Job drawing, mm, ordinate dimensions from the low corner. One solid piece. Give positions to 0.01 mm unless a question says otherwise; leave off trailing zeros. Loops run counter-clockwise (first coordinate to the right, second up) from the corner with the lowest first, then second, coordinate; pieces in that order, holes last. Notation, with made-up numbers: M 30,26.25 L 53,26.25 A8 cw 53,39.25 Z; hole C -12,-1 d2. An arc over 180 degrees is marked long. Answer in a Markdown table with one row per item.
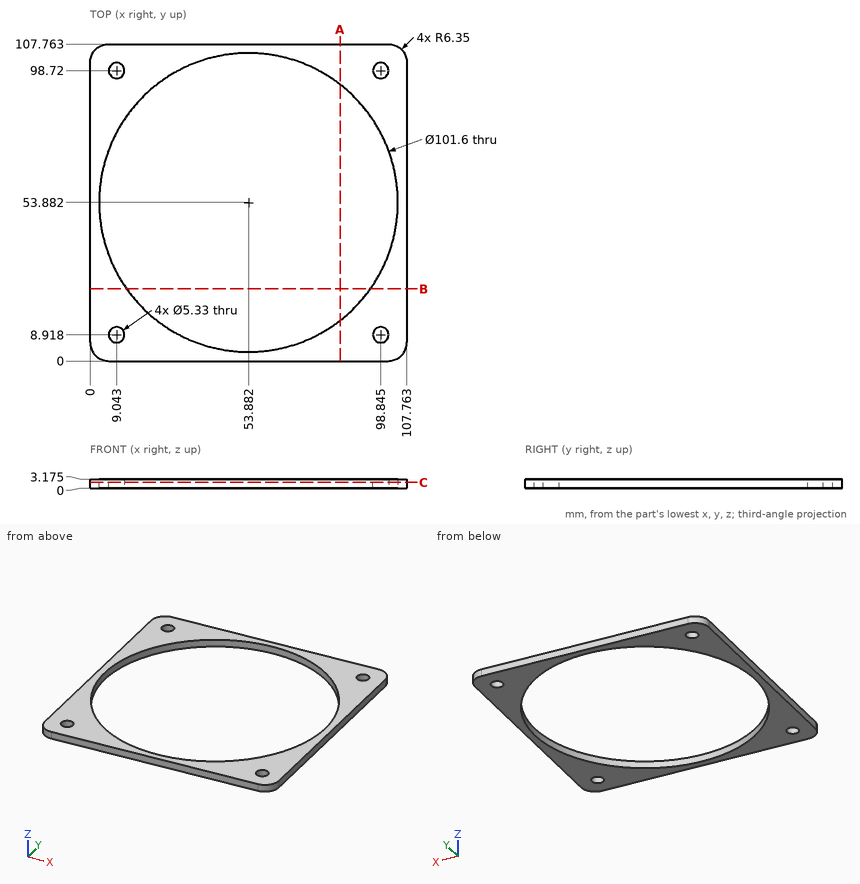
(1) Pin check, flat tip, straight feed: pin 1 Ø4.5 at (x, y) = (98.85, 98.72) entering from -Z. Stop position of the tip, or through.
Recorded:
| item | result |
|---|---|
| pin 1 | passes through |
(2) Drill centre lines: line 1 along Y through (x, z) = (53, 1); line 2 along Y through (x, z) = (17.5, 2.5) (1 decimal); line 3 along X through (y, z) = (37.5, 1.95) (1 decimal). Where is each one in solid material? Low to high.
Recorded:
| item | result |
|---|---|
| line 1 | y = 0 to 3.09, 104.67 to 107.76 |
| line 2 | y = 0 to 18.4, 89.3 to 107.8 |
| line 3 | x = 0 to 5.8, 102 to 107.8 |
(3) Saw through at A-A (x = 85). Write the cut outline in (y, z) (1 decimal).
Recorded:
| item | result |
|---|---|
| outline | M 0,0 L 13.7,0 L 13.7,3.2 L 0,3.2 Z; M 94,0 L 107.8,0 L 107.8,3.2 L 94,3.2 Z |
(4) Saw through at B-B (y = 24.5). Write the cut outline in (x, z) (1 decimal).
Recorded:
| item | result |
|---|---|
| outline | M 0,0 L 12.4,0 L 12.4,3.2 L 0,3.2 Z; M 95.3,0 L 107.8,0 L 107.8,3.2 L 95.3,3.2 Z |
(5) Saw through at C-C (z = 2.05). Give the number of separate pieces and of enclosed holes in the cut face, plus the area to 3 significant figures.
Recorded:
| item | result |
|---|---|
| separate pieces | 1 |
| enclosed holes | 5 |
| area | 3,380 mm^2 |
